Work out the finished part from the listing and answer in its coordinate system (mm). A direction names the side the tool comes from. Give positions to 0.01 mm unless a question says otherwise; leave off trailing zeros.
```python
from build123d import *

# Parameters (mm, degrees)
SKETCH_1_W                         = 12
SKETCH_1_H                         = 8
EXTRUDE_1_DEPTH                    = 150
CUT_EXTRUDE_1_DEPTH                = 151
CHAMFER_1_SIZE                     = 0.5
PATTERN_LINEAR_1_COUNT             = 4
PATTERN_LINEAR_1_PITCH             = 40
CHAMFER_1_OF_PATTERN_LINEAR_1_SIZE = 0.5
CHAMFER_2_SIZE                     = 0.3


with BuildPart() as part:
    # Эскиз1 → Бобышка-Вытянуть1 (new body)
    with BuildSketch(Plane(origin=(0, 0, 0), x_dir=(1, 0, 0), z_dir=(0, 1, 0))):
        with Locations((6, 4)):
            Rectangle(SKETCH_1_W, SKETCH_1_H)
    extrude(amount=EXTRUDE_1_DEPTH)

    # Эскиз2 → Вырез-Вытянуть1 (cut, through all)
    with BuildSketch(Plane(origin=(0, 150, 0), x_dir=(1, 0, 0), z_dir=(0, 1, 0))):
        with BuildLine():
            Line((11, 2.25), (11, 1.75))
            Line((11, 1.75), (11.5, 1.75))
            ThreePointArc((11.5, 1.75), (11.706107374, 1.524471742), (12, 1.440983006))
            Line((12, 1.440983006), (12, 2.559016994))
            ThreePointArc((12, 2.559016994), (11.706107374, 2.475528258), (11.5, 2.25))
            Line((11.5, 2.25), (11, 2.25))
        make_face()
    cut_extrude_1 = extrude(amount=-CUT_EXTRUDE_1_DEPTH, mode=Mode.SUBTRACT)

    # Зеркальное отражение1: Вырез-Вытянуть1 across plane
    add(cut_extrude_1.mirror(Plane(origin=(6, 0, 0), x_dir=(0, 0, 1), z_dir=(1, 0, 0))), mode=Mode.SUBTRACT)

    # Эскиз4 → Вырез-Повернуть1 (revolve, cut)
    with BuildSketch(Plane(origin=(6, 0, 0), x_dir=(0, 0, -1), z_dir=(1, 0, 0))):
        Polygon((0, 139), (4.5, 139), (4.5, 137.25), (8, 137.25), (8, 135), (0, 135), align=None)
    cut_revolve_1 = revolve(axis=Axis((6, 135, -8), (0, 0, 1)), mode=Mode.SUBTRACT)

    # Фаска1
    chamfer_1_edges = [part.edges().sort_by_distance(p)[0] for p in [
        (6, 131, 0),
        (6, 132.75, -8),
    ]]
    chamfer(chamfer_1_edges, length=CHAMFER_1_SIZE)

    # Линейный массив1: Вырез-Повернуть1 ×4
    with Locations(*[(0, -i * PATTERN_LINEAR_1_PITCH, 0) for i in range(1, PATTERN_LINEAR_1_COUNT)]):
        add(cut_revolve_1, mode=Mode.SUBTRACT)

    # Фаска1 of Линейный массив1
    chamfer_1_of_pattern_linear_1_edges = [part.edges().sort_by_distance(p)[0] for p in [
        (6, 91, 0),
        (6, 92.75, -8),
        (6, 51, 0),
        (6, 52.75, -8),
        (6, 11, 0),
        (6, 12.75, -8),
    ]]
    chamfer(chamfer_1_of_pattern_linear_1_edges, length=CHAMFER_1_OF_PATTERN_LINEAR_1_SIZE)

    # Фаска2
    chamfer_2_edges = [part.edges().sort_by_distance(p)[0] for p in [
        (12, 150, -0.720491503),
        (6, 150, -8),
        (12, 0, -5.279508497),
        (12, 150, -5.279508497),
        (11.25, 0, -2.25),
        (11.706107374, 0, -2.475528258),
        (11.706107374, 0, -1.524471742),
        (11.25, 0, -1.75),
        (11, 0, -2),
        (11.25, 150, -2.25),
        (11, 150, -2),
        (11.25, 150, -1.75),
        (11.706107374, 150, -1.524471742),
        (11.706107374, 150, -2.475528258),
        (0, 0, -0.720491503),
        (0, 150, -0.720491503),
        (0, 150, -5.279508497),
        (0.75, 150, -2.25),
        (1, 150, -2),
        (0.75, 150, -1.75),
        (0.293892626, 150, -1.524471742),
        (0.293892626, 150, -2.475528258),
        (0.75, 0, -2.25),
        (6, 0, -8),
        (1, 0, -2),
        (0.75, 0, -1.75),
        (0.293892626, 0, -1.524471742),
        (0.293892626, 0, -2.475528258),
        (12, 0, -0.720491503),
        (6, 0, 0),
        (0, 0, -5.279508497),
        (6, 150, 0),
        (0, 75, -8),
        (12, 75, -8),
        (12, 75, 0),
        (0, 75, 0),
    ]]
    chamfer(chamfer_2_edges, length=CHAMFER_2_SIZE)


solid = part.part
```
1. Straight lines are drawn through the part: probe 1 along Y at (x, z) = (6, -1.85); probe 2 along Z at (x, y) = (11.25, 34.5). For each, find the intervals that lie inside material, in ascending order.
Findings below:
probe 1: y = 0 to 11, 19 to 51, 59 to 91, 99 to 131, 139 to 150
probe 2: z = -8 to -2.25, -1.75 to 0
2. Which of the six approach directions +Z, -Z, +X, -X, +Y, -Y give full straight-line access (tool end or side, diameter ignored) to faces 1 (the face through (6, 74, 0)), 2 (the face through (4.799, 58.815, -2.528))?
Findings below:
face 1: +Z, +X, -X, +Y, -Y
face 2: +Z
3. The mould has two halves that part along X. Classify faces 3 (the face through (0, 74, -5)), 4 (the face through (9.905, 94.133, -2.528)), 5 (the face through (6, 0, -4)), 6 (the face through (9.905, 134.133, -2.528)): pulls with the +X half, pulls with the -X half, needs draft (parallel to the pull), parting line crosses it, or undercut.
Findings below:
face 3: pulls with the -X half
face 4: undercut
face 5: needs draft
face 6: undercut
4. Given P1, Ø5, axis at x = 6, y = 55, coming from the +Z side; P2, Ø3.5, axis at x = 6, y = 135, coming from the -Z side; P3, Ø5, axis at x = 6, y = 15, coming from the -Z side; P4, Ø0.6, axis at y = 100.5, z = -2, coming from the -X side, each flat-ended and moving along its own axis, determine where each tip first touches the part or whether it passes through.
Findings below:
P1: stops at z = -4.5
P2: passes through
P3: stops at z = -7.75
P4: stops at x = 0.47
